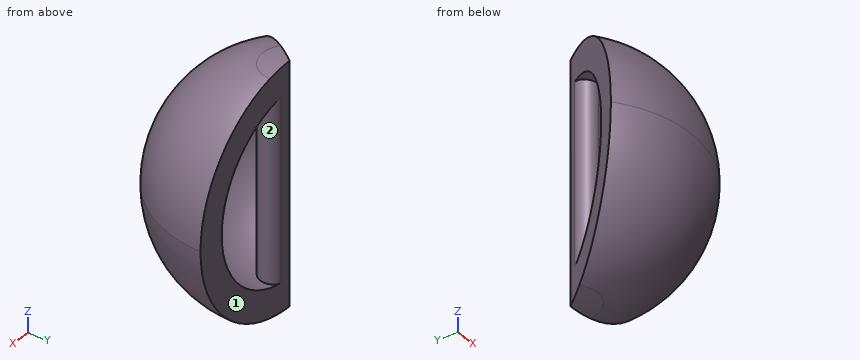
```python
from build123d import *

# Parameters (mm, degrees)
F1_ANGLE = 127.6370568736
F2_R     = 2


with BuildPart() as f1:
    # F0 (on Front) → F1 (revolve)
    with BuildSketch(Plane.XZ):
        with BuildLine():
            ThreePointArc((4.9959747121, 21.9383280283), (2.5137242653, 22.3591410908), (0, 22.5))
            Line((0, 22.5), (0, 17.1344819252))
            ThreePointArc((0, 17.1344819252), (2.525573198, 16.9473287236), (4.9959747121, 16.3899575204))
            Line((4.9959747121, 16.3899575204), (4.9959747121, 21.9383280283))
        make_face()
        with BuildLine():
            ThreePointArc((4.9959747121, 16.3899575204), (2.525573198, 16.9473287236), (0, 17.1344819252))
            Line((0, 17.1344819252), (0, -17.1344819252))
            ThreePointArc((0, -17.1344819252), (2.525573198, -16.9473287236), (4.9959747121, -16.3899575204))
            Line((4.9959747121, -16.3899575204), (4.9959747121, 16.3899575204))
        make_face()
        with BuildLine():
            Line((0, -17.1344819252), (0, -22.5))
            ThreePointArc((0, -22.5), (2.5137242653, -22.3591410908), (4.9959747121, -21.9383280283))
            Line((4.9959747121, -21.9383280283), (4.9959747121, -16.3899575204))
            ThreePointArc((4.9959747121, -16.3899575204), (2.525573198, -16.9473287236), (0, -17.1344819252))
        make_face()
        with BuildLine():
            ThreePointArc((22.5, 0), (17.5877717608, 14.0328288128), (4.9959747121, 21.9383280283))
            Line((4.9959747121, 21.9383280283), (4.9959747121, 16.3899575204))
            ThreePointArc((4.9959747121, 16.3899575204), (13.7694209981, 10.1977211288), (17.1344819252, 0))
            ThreePointArc((17.1344819252, 0), (13.7694209981, -10.1977211288), (4.9959747121, -16.3899575204))
            Line((4.9959747121, -16.3899575204), (4.9959747121, -21.9383280283))
            ThreePointArc((4.9959747121, -21.9383280283), (17.5877717608, -14.0328288128), (22.5, 0))
        make_face()
    revolve(axis=Axis((0, 0, 0), (0, 0, -1)), revolution_arc=F1_ANGLE)

    # F2
    f2_edges = [f1.edges().sort_by_distance(p)[0] for p in [
        (-3.050829, -3.956287, 0),
        (4.995975, 0, 0),
    ]]
    fillet(f2_edges, radius=F2_R)


solid = f1.part
```
The model under review builds one solid part; all positions refer to its coordinate system, in mm. Face numbers are marked on the shaded views. Give positions to 0.01 mm unless a question says otherwise; leave off trailing zeros. Write each loop counter-clockwise with the first axis right and the second up, starting at its lowest first coordinate (ties: lowest second). Pieces come first, ordered by that corner, then holes. Notation, with made-up numbers: (-22, -27.75) -> (15, -27.75) arc R22 ccw to (15, -6.75) -> close; hole circle Ø5 at (72.5, 50). An arc over 180 degrees is marked (long way). Put each result on its own line as item: value.
(1) We need section D-D, the plane x = -5. Give the boundary of the cut face in (y, z).
Results are:
outline: (-6.48, -20.96) -> (-6.48, -15.05) arc R16.39 cw to (-6.48, 15.05) -> (-6.48, 20.96) arc R21.94 ccw to start
(2) We need section C-C, the plane y = -15.25. Give the boundary of the cut face in (x, z), and give its area (3 significant figures).
Results are:
outline: (-11.76, -11.64) arc R16.54 ccw (long way) to (-11.76, 11.64) -> close; hole circle Ø15.62 at (0, 0)
area: 591 mm²
(3) To check wall thickness, follow probe 1 along Z at (x, y) = (6, -11.5); probe 2 along X at (y, z) = (-2, -7); probe 3 along Z at (x, y) = (8, -3). State the ranges of each line that lie inside material, in increasing order. Write a range as from..to.
Results are:
probe 1: -18.38..-11.2, 11.2..18.38
probe 2: -1.52..4.23, 15.51..21.29
probe 3: -20.81..-14.85, 14.85..20.81
(4) We need section A-A, the plane z = 14.5. Give the boundary of the cut face in (x, y).
Results are:
outline: (-10.51, -13.62) arc R17.2 ccw to (17.2, 0) -> (9.13, 0) arc R9.13 cw to (-5.57, -7.23) -> close; (-1.36, -1.77) arc R2 ccw to (0.37, -4.98) arc R5 ccw to (3.72, -3.34) arc R2 ccw to (2.23, 0) -> (0, 0) -> close
(5) The part is to be moulded in two halves that separate along Z. For the marked faces 1 and 2, say which applies: pulls with the +Z half, pulls with the -Z half, needs draft (parallel to the pull), parting line crosses it, or undercut.
Results are:
face 1: needs draft
face 2: undercut
(6) We need section B-B, the plane x = 1. Give the boundary of the cut face in (y, z).
Results are:
outline: (0, -22.48) -> (0, 22.48) arc R22.48 ccw to start; hole (-4.89, -16.39) -> (-4.89, 16.39) arc R17.11 ccw to start
(7) For pin 1 Ø6 at (x, z) = (18.5, -12.5) entering from +Y; pin 2 Ø12 at (y, z) = (-20, -13.5) entering from +X; pin 3 Ø10 at (y, z) = (-17.5, 16.5) entering from -X; pin 4 Ø12 at (x, y) = (-2, -16.5) entering from +Z, all flat-tipped, find the tip position at first contact; note any pin that passes through.
Results are:
pin 1: y = 0
pin 2: x = 13.33
pin 3: x = -11.55
pin 4: z = 19.84
